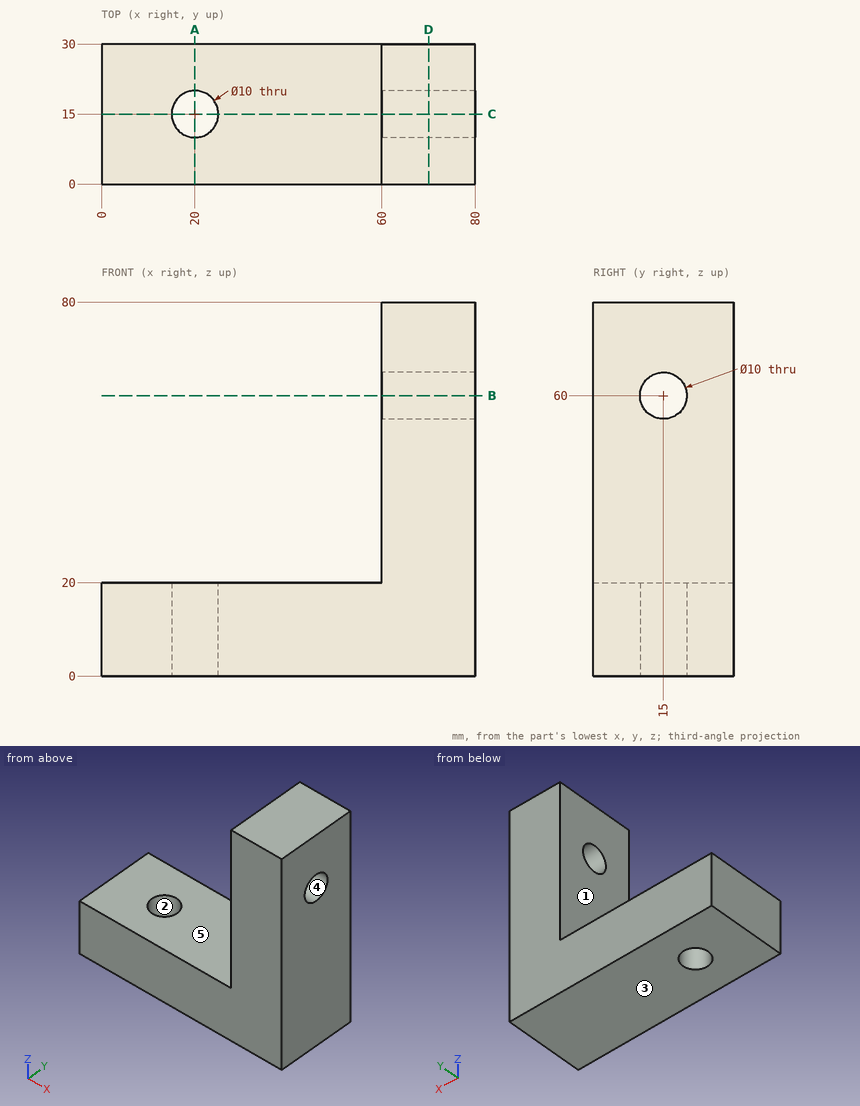
Input: dimensioned drawing with shaded views. Units: mm. Origin: part minimum x, y, z. A direction names the side the tool comes from. Give positions to 0.01 mm unless a question says otherwise; leave off trailing zeros. Write each loop counter-clockwise with the first axis right and the second up, starting at its lowest first coordinate (ties: lowest second). Pieces come first, ordered by that corner, then holes. Notation, with made-up numbers: M -5,-37 L 0,-37 A10 cw 0,-27 Z; hole C 19.25,-33.5 d7. An arc over 180 degrees is marked long. Write item = value, one per line. Start each with the question number.
1) Reachability of the marked faces 4 and 5 from +Z, -Z, +X, -X, +Y, -Y: full face, straight path, thin tool, end or side. Return the list, or none.
2) Cut plane C-C on y = 15. Return the cut outline in (x, z).
3) First-contact query: pin 1 Ø16 at (y, z) = (15, 60) entering from +X. Flat tip, straight axial feed; report the tip coordinate or a pass-through.
4) Cut plane D-D on x = 70. Return the cut outline in (y, z), then the cut area to 3 significant figures.
5) Draft query along X for the marked faces 1, 2 and 3. Return one class per face: +X half, -X half, draft (parallel to the pull), parting line (faces both ways), or undercut.
6) Cut plane B-B on z = 60. Return the cut outline in (x, y), then the cut area to 3 significant figures.
7) Cut plane A-A on x = 20. Return the cut outline in (y, z), then the cut area to 3 significant figures.
8) Material intervals for line 1 along Z through (x, y) = (66, 15); line 2 along Y through (x, z) = (20, 13.5); line 3 along Z through (x, y) = (54.5, 19.5), sorted ascending. Write a range as [from, to].
Solved:
q1.face_4 = +X, -X
q1.face_5 = +Z, -X, +Y, -Y
q2.outline = M 0,0 L 15,0 L 15,20 L 0,20 Z; M 25,0 L 80,0 L 80,55 L 60,55 L 60,20 L 25,20 Z; M 60,65 L 80,65 L 80,80 L 60,80 Z
q3.pin_1 = 80
q4.outline = M 0,0 L 30,0 L 30,80 L 0,80 Z; hole C 15,60 d10
q4.area = 2,320 mm2
q5.face_1 = -X half
q5.face_2 = undercut
q5.face_3 = draft
q6.outline = M 60,0 L 80,0 L 80,10 L 60,10 Z; M 60,20 L 80,20 L 80,30 L 60,30 Z
q6.area = 400 mm2
q7.outline = M 0,0 L 10,0 L 10,20 L 0,20 Z; M 20,0 L 30,0 L 30,20 L 20,20 Z
q7.area = 400 mm2
q8.line_1 = [0, 55], [65, 80]
q8.line_2 = [0, 10], [20, 30]
q8.line_3 = [0, 20]
